```python
from build123d import *

# Parameters (mm, degrees)
ESQUISSE2_R             = 30
BOSS_EXTRU_1_DEPTH      = 3
ENL_V_MAT_EXTRU_1_DEPTH = 43.532340636
BOSS_EXTRU_3_START      = 6
ESQUISSE5_W             = 10.501413836
ESQUISSE5_H             = 10.144569676
BOSS_EXTRU_3_DEPTH      = 6
ESQUISSE8_R             = 28.75
BOSS_EXTRU_4_DEPTH      = 1.5
BOSS_EXTRU_5_START      = 3
ESQUISSE9_R             = 30
BOSS_EXTRU_5_DEPTH      = 3
ENL_V_MAT_EXTRU_4_DEPTH = 44.370496884
CONG_1_R                = 3
CONG_2_R                = 2


with BuildPart() as part:
    # Esquisse2 → Boss.-Extru.1 (new body)
    with BuildSketch(Plane.XY):
        Circle(ESQUISSE2_R)
    extrude(amount=BOSS_EXTRU_1_DEPTH)

    # Esquisse4 → Enlèv. mat.-Extru.1 (cut, through all)
    with BuildSketch(Plane.XY.offset(3)):
        with BuildLine():
            Line((-2.1, -1.8), (2.1, -1.8))
            ThreePointArc((2.1, -1.8), (2.765863337, 0), (2.1, 1.8))
            Line((2.1, 1.8), (-2.1, 1.8))
            ThreePointArc((-2.1, 1.8), (-2.765863337, 0), (-2.1, -1.8))
        make_face()
    extrude(amount=-ENL_V_MAT_EXTRU_1_DEPTH, mode=Mode.SUBTRACT)

    # Esquisse5 → Boss.-Extru.3 (add)
    with BuildSketch(Plane.XY.offset(3).offset(BOSS_EXTRU_3_START)):
        Rectangle(ESQUISSE5_W, ESQUISSE5_H)
        with BuildLine():
            Line((-2.1, 1.8), (2.1, 1.8))
            ThreePointArc((2.1, 1.8), (2.765863337, 0), (2.1, -1.8))
            Line((2.1, -1.8), (-2.1, -1.8))
            ThreePointArc((-2.1, -1.8), (-2.765863337, 0), (-2.1, 1.8))
        make_face(mode=Mode.SUBTRACT)
    extrude(amount=-BOSS_EXTRU_3_DEPTH)

    # Esquisse8 → Boss.-Extru.4 (add)
    with BuildSketch(Plane(origin=(0, 0, 0), x_dir=(-1, 0, 0), z_dir=(0, 0, -1))):
        Circle(ESQUISSE8_R)
    extrude(amount=BOSS_EXTRU_4_DEPTH)

    # Esquisse9 → Boss.-Extru.5 (add)
    with BuildSketch(Plane(origin=(0, 0, -1.5), x_dir=(-1, 0, 0), z_dir=(0, 0, -1)).offset(BOSS_EXTRU_5_START)):
        with Locations(Location((0, 0, 0), (0, 0, 180))):
            Circle(ESQUISSE9_R)
    extrude(amount=-BOSS_EXTRU_5_DEPTH)

    # Esquisse10 → Enlèv. mat.-Extru.4 (cut, through all)
    with BuildSketch(Plane.XY):
        with BuildLine():
            Line((-2.1, 1.8), (2.1, 1.8))
            ThreePointArc((2.1, 1.8), (2.765863337, 0), (2.1, -1.8))
            Line((2.1, -1.8), (-2.1, -1.8))
            ThreePointArc((-2.1, -1.8), (-2.765863337, 0), (-2.1, 1.8))
        make_face()
    extrude(amount=-ENL_V_MAT_EXTRU_4_DEPTH, mode=Mode.SUBTRACT)

    # Congé1
    # the kernel refuses this fillet: 3 mm, written as the material it takes off along each edge
    with BuildSketch(Plane(origin=(-2.250706918, -2.072284838, 6), x_dir=(-1, 0, 0), z_dir=(0, -1, 0))) as cong_1_piece_1_section:
        Polygon((0, 0), (CONG_1_R, 0), (CONG_1_R, -CONG_1_R), (0, -CONG_1_R), align=None)
    cong_1_piece_1 = extrude(amount=CONG_1_R, mode=Mode.PRIVATE)
    cong_1_piece_1 = cong_1_piece_1 - Plane(origin=(-2.250706918, -2.072284838, 6), x_dir=(0.7071067811865475, 0, -0.7071067811865475), z_dir=(0, -1, 0)) * Sphere(CONG_1_R, mode=Mode.PRIVATE)
    add(cong_1_piece_1, mode=Mode.SUBTRACT)
    with BuildSketch(Plane(origin=(-2.250706918, 2.072284838, 6), x_dir=(-1, 0, 0), z_dir=(0, 1, 0))) as cong_1_piece_2_section:
        Polygon((0, 0), (CONG_1_R, 0), (CONG_1_R, CONG_1_R), (0, CONG_1_R), align=None)
    cong_1_piece_2 = extrude(amount=CONG_1_R, mode=Mode.PRIVATE)
    cong_1_piece_2 = cong_1_piece_2 - Plane(origin=(-2.250706918, 2.072284838, 6), x_dir=(0.7071067811865475, 0, -0.7071067811865475), z_dir=(0, 1, 0)) * Sphere(CONG_1_R, mode=Mode.PRIVATE)
    add(cong_1_piece_2, mode=Mode.SUBTRACT)
    with BuildSketch(Plane(origin=(2.250706918, -2.072284838, 6), x_dir=(0, -1, 0), z_dir=(1, 0, 0))) as cong_1_piece_3_section:
        Polygon((0, 0), (CONG_1_R, 0), (CONG_1_R, -CONG_1_R), (0, -CONG_1_R), align=None)
    cong_1_piece_3 = extrude(amount=CONG_1_R, mode=Mode.PRIVATE)
    cong_1_piece_3 = cong_1_piece_3 - Plane(origin=(2.250706918, -2.072284838, 6), x_dir=(0, 0.7071067811865475, -0.7071067811865475), z_dir=(1, 0, 0)) * Sphere(CONG_1_R, mode=Mode.PRIVATE)
    add(cong_1_piece_3, mode=Mode.SUBTRACT)
    with BuildSketch(Plane(origin=(2.250706918, 2.072284838, 6), x_dir=(1, 0, 0), z_dir=(0, 1, 0))) as cong_1_piece_4_section:
        Polygon((0, 0), (CONG_1_R, 0), (CONG_1_R, -CONG_1_R), (0, -CONG_1_R), align=None)
    cong_1_piece_4 = extrude(amount=CONG_1_R, mode=Mode.PRIVATE)
    cong_1_piece_4 = cong_1_piece_4 - Plane(origin=(2.250706918, 2.072284838, 6), x_dir=(-0.7071067811865475, 0, -0.7071067811865475), z_dir=(0, 1, 0)) * Sphere(CONG_1_R, mode=Mode.PRIVATE)
    add(cong_1_piece_4, mode=Mode.SUBTRACT)
    with BuildSketch(Plane(origin=(-5.250706918, -2.072284838, 9), x_dir=(0, 0, -1), z_dir=(0, 1, 0))) as cong_1_piece_5:
        with BuildLine():
            CenterArc((CONG_1_R, -CONG_1_R), CONG_1_R, 90, 90)
            Line((0, -CONG_1_R), (0, 0))
            Line((0, 0), (CONG_1_R, 0))
        make_face()
    extrude(amount=4.144569676, mode=Mode.SUBTRACT)
    with BuildSketch(Plane(origin=(-5.250706918, 5.072284838, 6), x_dir=(0, -1, 0), z_dir=(0, 0, -1)), Plane(origin=(5.250706918, -5.072284838, 6), x_dir=(0, 1, 0), z_dir=(0, 0, -1)), Plane(origin=(5.250706918, 5.072284838, 6), x_dir=(-1, 0, 0), z_dir=(0, 0, -1))) as cong_1_piece_6:
        with BuildLine():
            CenterArc((CONG_1_R, -CONG_1_R), CONG_1_R, 90, 90)
            Line((0, -CONG_1_R), (0, 0))
            Line((0, 0), (CONG_1_R, 0))
        make_face()
    extrude(amount=3, mode=Mode.SUBTRACT)
    with BuildSketch(Plane(origin=(2.250706918, -5.072284838, 9), x_dir=(0, 1, 0), z_dir=(-1, 0, 0)), Plane(origin=(-2.250706918, 5.072284838, 9), x_dir=(0, -1, 0), z_dir=(1, 0, 0))) as cong_1_piece_7:
        with BuildLine():
            CenterArc((CONG_1_R, CONG_1_R), CONG_1_R, 180, 90)
            Line((0, CONG_1_R), (0, 0))
            Line((0, 0), (CONG_1_R, 0))
        make_face()
    extrude(amount=4.501413836, mode=Mode.SUBTRACT)
    with BuildSketch(Plane(origin=(-5.250706918, -5.072284838, 6), x_dir=(0, 1, 0), z_dir=(0, 0, -1))) as cong_1_piece_8:
        with BuildLine():
            CenterArc((CONG_1_R, CONG_1_R), CONG_1_R, 180, 90)
            Line((0, CONG_1_R), (0, 0))
            Line((0, 0), (CONG_1_R, 0))
        make_face()
    extrude(amount=3, mode=Mode.SUBTRACT)
    with BuildSketch(Plane(origin=(5.250706918, 2.072284838, 9), x_dir=(-1, 0, 0), z_dir=(0, -1, 0))) as cong_1_piece_9:
        with BuildLine():
            CenterArc((CONG_1_R, CONG_1_R), CONG_1_R, 180, 90)
            Line((0, CONG_1_R), (0, 0))
            Line((0, 0), (CONG_1_R, 0))
        make_face()
    extrude(amount=4.144569676, mode=Mode.SUBTRACT)

    # Congé2
    cong_2_edges = [part.edges().sort_by_distance(p)[0] for p in [
        (-5.250706918, 0, 3),
        (0, 5.072284838, 3),
        (0, -5.072284838, 3),
        (5.250706918, 0, 3),
        (-4.372027261, 4.193605182, 3),
        (-4.372027261, -4.193605182, 3),
        (4.372027261, -4.193605182, 3),
        (4.372027261, 4.193605182, 3),
    ]]
    fillet(cong_2_edges, radius=CONG_2_R)


solid = part.part
```
Here's how the part is built. I have some questions about the finished solid (model axes, mm). A direction names the side the tool comes from. Coordinates: 2 decimals unless noted, no trailing zeros. Order: outer loops, then holes, each group sorted by start corner. A loop starts at its lowest first (then second) coordinate and runs counter-clockwise, first axis right, second up.
1) Imagine slicing it at B-B on y = 0. List the corners of the cut face in (x, z) for me, and give its area (3 significant figures).
2) We'd pull the mould along Z, two halves only. Please class faces 1 (the face through (2, 29, -1.5)), 2 (the face through (0.032, -4.217, 8.098)), 3 (the face through (-2.766, -0.027, 2.344)): +Z half, -Z half, draft (parallel to the pull), parting line (faces both ways), or undercut.
3) I need wall thicknesses on line 1 (Z direction, x = -13, y = 27); line 2 (Z direction, x = -15, y = 15); line 3 (Y direction, x = -1.5, z = 5.5). Which ranges of each line are inside material? Lowest first, please.
4) Will these pins go through, and if not, where does the flat tip stop? pin 1 (6 mm diameter, centred on x = 17.5, z = 5, fed in from +Y); pin 2 (1.5 mm diameter, centred on y = 21.5, z = 1.5, fed in from -X); pin 3 (10 mm diameter, centred on x = -11, y = -18, fed in from +Z).
5) Imagine slicing it at D-D on x = -25. List the corners of the cut face in (y, z) for me, and give its area (3 significant figures).
6) Imagine slicing it at A-A on x = 0. List the corners of the cut face in (y, z) for me.
7) Imagine slicing it at C-C on z = 4.25. List the corners of the cut face in (x, y) for me.
8) Which directions (+Z, -Z, +X, -X, +Y, -Y) give clear straight access to the entire face, cutting with the end or side of a thin tool? Please do faces 4 (the face through (0, 1.8, 2)), 5 (the face through (4.349, 4.217, 5.507)), 6 (the face through (-4.349, -4.217, 5.507)).
Response values:
1. outline: (-30, -4.5) - (-2.77, -4.5) - (-2.77, 8.96) arc R3 ccw to (-5.25, 6) - (-5.25, 5) arc R2 cw to (-7.25, 3) - (-30, 3) - (-30, 0) - (-28.75, 0) - (-28.75, -1.5) - (-30, -1.5) - close; (2.77, -4.5) - (30, -4.5) - (30, -1.5) - (28.75, -1.5) - (28.75, 0) - (30, 0) - (30, 3) - (7.25, 3) arc R2 cw to (5.25, 5) - (5.25, 6) arc R3 ccw to (2.77, 8.96) - close
1. area: 432 mm2
2. face 1: undercut
2. face 2: +Z half
2. face 3: draft
3. line 1: z = -4.5 to -1.5, 0 to 3
3. line 2: z = -4.5 to 3
3. line 3: y = -5.07 to -1.8, 1.8 to 5.07
4. pin 1: stops at y = 25.83
4. pin 2: stops at x = -21.67
4. pin 3: stops at z = 3
5. outline: (-16.58, -4.5) - (16.58, -4.5) - (16.58, -1.5) - (14.2, -1.5) - (14.2, 0) - (16.58, 0) - (16.58, 3) - (-16.58, 3) - (-16.58, 0) - (-14.2, 0) - (-14.2, -1.5) - (-16.58, -1.5) - close
5. area: 242 mm2
6. outline: (-30, -4.5) - (-1.8, -4.5) - (-1.8, 9) - (-2.07, 9) arc R3 ccw to (-5.07, 6) - (-5.07, 5) arc R2 cw to (-7.07, 3) - (-30, 3) - (-30, 0) - (-28.75, 0) - (-28.75, -1.5) - (-30, -1.5) - close; (1.8, -4.5) - (30, -4.5) - (30, -1.5) - (28.75, -1.5) - (28.75, 0) - (30, 0) - (30, 3) - (7.07, 3) arc R2 cw to (5.07, 5) - (5.07, 6) arc R3 ccw to (2.07, 9) - (1.8, 9) - close
7. outline: (-5.4, -2.07) arc R3.15 ccw to (-2.25, -5.22) - (2.25, -5.22) arc R3.15 ccw to (5.4, -2.07) - (5.4, 2.07) arc R3.15 ccw to (2.25, 5.22) - (-2.25, 5.22) arc R3.15 ccw to (-5.4, 2.07) - close; hole (-2.1, -1.8) - (2.1, -1.8) arc R2.77 ccw to (2.1, 1.8) - (-2.1, 1.8) arc R2.77 ccw to start
8. face 4: +Z, -Z
8. face 5: +Z, +X, +Y
8. face 6: +Z, -X, -Y
